Autodesk Inventor part; units mm, degrees
ref_plane "YZ Plane" through (0, 0, 0) normal (1, 0, 0) x (0, 1, 0)
ref_plane "XZ Plane" through (0, 0, 0) normal (0, 1, 0) x (-1, 0, 0)
ref_plane "XY Plane" through (0, 0, 0) normal (0, 0, 1) x (1, 0, 0)
sketch "Sketch1" plane through (0, 0, 0) normal (0, 1, 0) x (-1, 0, 0)
  circle A0 centre (0, 0) radius 17.5
  dimension "d0" = 35
extrude "Base" add sketch "Sketch1" along normal blind 10
sketch "Sketch2" plane through (0, 10, 0) normal (0, 1, 0) x (1, 0, 0)
  circle A0 centre (0, 0) radius 8
  circle A1 centre (-8, 0) radius 0.8
  dimension "d3" = 16
  dimension "d4" = 1.6
extrude "Mounting Hole" cut sketch "Sketch2" against normal through all contours A1 A0 | A0 A1 picked at (-7.7304, 0) picked at (-8.2616, 0.0332)
pattern_circular "Circular Pattern1" count 8 over 360 about axis through (0, 0, 0) along (0, 1, 0) of "Mounting Hole"
sketch "Sketch3" plane through (0, 10, 0) normal (0, 1, 0) x (1, 0, 0)
  arc A0 (-16.6435, 5.4078) -> (-17.5, 0) centre (0, 0) ccw
  line L0 (0, 0) -> (-16.6435, 5.4078) construction
  line L1 (0, 0) -> (-17.5, 0) construction
  line L2 (0, 0) -> (-25.2614, 4.001)
  line L3 (0, 0) -> (25.5763, 0) construction
  line L4 (-17.5, 0) -> (-21.2042, 3.3584)
  line L5 (-16.6435, 5.4078) -> (-21.2042, 3.3584)
  dimension "d11" = 18
  dimension "d12" = 171
  dimension "d13" = 5
extrude "Gear Tooth" add sketch "Sketch3" against normal blind 10
pattern_circular "Circular Pattern2" count 20 over 360 about axis through (0, 0, 0) along (0, 1, 0) of "Gear Tooth"
sketch "Sketch6" plane through (0, 10, 0) normal (0, 1, 0) x (1, 0, 0)
  point P0 (0, 0)
sketch "Sketch7" plane through (0, 10, 0) normal (0, 1, 0) x (1, 0, 0)
  circle A0 centre (0, 0) radius 10
  dimension "d26" = 20
extrude "Extrusion6" cut sketch "Sketch7" against normal blind 2
sketch "Sketch8" plane through (0, 8, 0) normal (0, 1, 0) x (1, 0, 0)
  circle A0 centre (0, 0) radius 4
  dimension "d29" = 8
extrude "Extrusion7" cut sketch "Sketch8" against normal blind 1.9
sketch "Sketch9" plane through (0, 6.1, 0) normal (0, 1, 0) x (1, 0, 0)
  circle A0 centre (0, 0) radius 2.25
  dimension "d32" = 4.5
extrude "Extrusion8" cut sketch "Sketch9" against normal blind 2.5
sketch "Sketch10" plane through (0, 10, 0) normal (0, 1, 0) x (1, 0, 0)
  circle A0 centre (0, 0) radius 10
extrude "Extrusion9" add sketch "Sketch10" against normal blind 10
properties part number "BarMountSmallGear"
Part model, mm, in its own coordinate system. A direction names the side the tool comes from. Round coordinates to 2 decimals unless told otherwise and drop trailing zeros. Write each loop counter-clockwise with the first axis right and the second up, starting at its lowest first coordinate (ties: lowest second). Pieces come first, ordered by that corner, then holes. Notation, with made-up numbers: M 15.5,-11.5 L 35.5,-11.5 A21 cw 35.5,13.5 Z; hole C 51.25,-9.5 d6. An arc over 180 degrees is marked long. One line per question, with ' | ' between items.
(1) Saw through at D-D on z = 1. Write the cut outline in (x, y).
Answer key:
outline: M -18.6,0 L 18.6,0 L 18.6,10 L -18.6,10 Z
(2) 3-axis set-ups, long thin cutter, end or side, ignore diameter. For faces 4 (the face through (19.33, 5.07, 1.66)), 5 (the face through (0, 0, 0)), 6 (the face through (-12.699, 5.07, 14.662)), 7 (the face through (-17.87, 5.07, -7.55)), 8 (the face through (7.55, 5.07, -17.87)): which of +Z, -Z, +X, -X, +Y, -Y reach the whole face in a straight line?
Answer key:
face 4: +X, +Y, -Y | face 5: +Z, -Z, +X, -X, -Y | face 6: +Z, +Y, -Y | face 7: -X, +Y, -Y | face 8: -Z, +Y, -Y
(3) Saw through at A-A on z = -18. Write the cut outline in (x, y), then the cut area to 3 significant figures.
Answer key:
outline: M -9.87,0 L -7.78,0 L -7.78,10 L -9.87,10 Z; M -4.8,0 L -0.45,0 L -0.45,10 L -4.8,10 Z; M 0.45,0 L 4.8,0 L 4.8,10 L 0.45,10 Z; M 7.78,0 L 9.87,0 L 9.87,10 L 7.78,10 Z | area: 129 mm^2
(4) Saw through at C-C on x = -6. Write the cut outline in (y, z), then the cut area to 3 significant figures.
Answer key:
outline: M 0,-16.98 L 10,-16.98 L 10,16.98 L 0,16.98 Z | area: 340 mm^2
(5) Saw through at B-B on x = 18.5. Write the cut outline in (y, z), then the cut area to 3 significant figures.
Answer key:
outline: M 0,-9.81 L 10,-9.81 L 10,-8.65 L 0,-8.65 Z; M 0,-4.57 L 10,-4.57 L 10,-0.91 L 0,-0.91 Z; M 0,0.91 L 10,0.91 L 10,4.57 L 0,4.57 Z; M 0,8.65 L 10,8.65 L 10,9.81 L 0,9.81 Z | area: 96.7 mm^2
(6) Probe line 1 along Z through (x, y) = (19.5, 2.75); line 2 along X through (y, z) = (7, 4.5); line 3 along X through (y, z) = (8.5, -13). List the from-to ranges inside material, lowest first.
Answer key:
line 1: z = -4.12 to -1.81, 1.81 to 4.12 | line 2: x = -18.66 to 18.66 | line 3: x = -14.72 to 14.72
(7) Pin check, flat tips, straight feed: pin 1 (4 mm diameter, centred on y = 3, z = 15.5, fed in from +X); pin 2 (6 mm diameter, centred on y = 6, z = 0.5, fed in from +X); pin 3 (5 mm diameter, centred on x = -16, y = 1.5, fed in from +Z). Stop position of each tip, or through.
Answer key:
pin 1: stops at x = 15.18 | pin 2: stops at x = 21.2 | pin 3: stops at z = 15.18
(8) Two-plate mould, pull along X, no slides. Class faces 1 (the face through (4.4, 5.07, 18.89)), 2 (the face through (14.662, 5.07, -12.699)), 3 (the face through (0, 10, 0)): released by +X, released by -X, zero draft, split by the parting line, or undercut.
Answer key:
face 1: undercut | face 2: released by +X | face 3: zero draft
